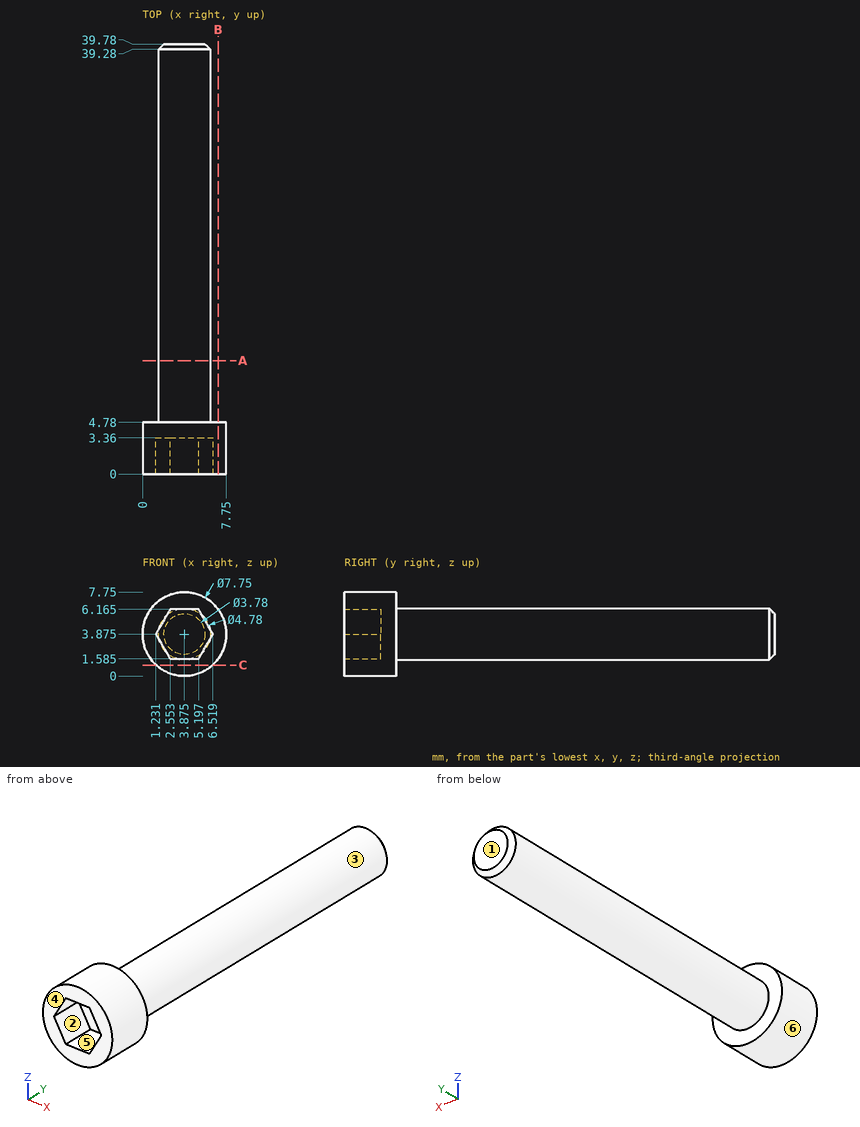
Drawing for the job (mm, zero at the part's lowest x, y, z). A direction names the side the tool comes from. Give positions to 0.01 mm unless a question says otherwise; leave off trailing zeros. Loops run counter-clockwise (first coordinate to the right, second up) from the corner with the lowest first, then second, coordinate; pieces in that order, holes last.
Item 1: Drill centre lines: line 1 along Y through (x, z) = (2.5, 1); line 2 along Y through (x, z) = (4.5, 3); line 3 along X through (y, z) = (16.5, 4). Where is each one in solid material? Low to high.
Check values:
line 1: y = 0 to 4.78
line 2: y = 3.36 to 39.78
line 3: x = 1.49 to 6.26
Item 2: Mould opens along X. For the marked faces 4, 5 and 6 say: +X half, -X half, draft (parallel to the pull), parting line (faces both ways), or undercut.
Check values:
face 4: draft
face 5: undercut
face 6: parting line
Item 3: Slice it at B-B (x = 7). Write the cut outline in (y, z).
Check values:
outline: (0, 1.58) - (4.78, 1.58) - (4.78, 6.17) - (0, 6.17) - close
Item 4: Which spindle directions (+Z, -Z, +X, -X, +Y, -Y) get a long thin tool onto all of the face, cutting with end or side? Do the marked faces 1, 2 and 3. Say none if no direction does.
Check values:
face 1: +Z, -Z, +X, -X, +Y
face 2: -Y
face 3: +Y
Item 5: Drop flat-ended pins along their axis: P1, Ø4, axis at y = 32.5, z = 7, coming from the -X side; P2, Ø2.5, axis at x = 4.5, z = 4.5, coming from the -Y side. Give the stop position or say it passes through.
Check values:
P1: stops at x = 1.77
P2: stops at y = 3.36
Item 6: Slice it at A-A (y = 10.5). Write the cut outline in (x, z) (1 decimal).
Check values:
outline: circle Ø4.8 at (3.9, 3.9)
Item 7: Slice it at C-C (z = 1). Write the cut outline in (x, y).
Check values:
outline: (1.28, 0) - (6.47, 0) - (6.47, 4.78) - (1.28, 4.78) - close
